Part model, mm, in its own coordinate system. Round coordinates to 2 decimals unless told otherwise and drop trailing zeros. Loops run counter-clockwise (first coordinate to the right, second up) from the corner with the lowest first, then second, coordinate; pieces in that order, holes last. Notation, with made-up numbers: M 44,42.25 L 67,42.25 A22 cw 67,62.25 Z; hole C -5,-18.5 d10. An arc over 180 degrees is marked long. Put each result on its own line as item: value. Start each with the question number.
1) Slice it at C-C on y = 155. Give the cut face in (x, z), then the cut area to 3 significant figures.
2) Probe line 1 along Y through (x, z) = (209, -2.25); line 2 along Y through (x, z) = (207.5, -1); line 3 along X through (y, z) = (99, 2.5). List the from-to ranges inside material, lowest first.
3) Pull direction X, two halves, no side cores. Call faces 1 (the cylindrical face through (212.715, 153.411, -0.07)), 2 (the cylindrical face through (215.896, 139.327, 0.07)), 3 (the flat face through (209, 140, -5)): +X half, -X half, draft (parallel to the pull), parting line (faces both ways), or undercut.
4) Slice it at D-D on y = 135.5. Give the cut face in (x, z), then the cut area to 3 significant figures.
5) Slice it at B-B on x = 208.5. Give the cut face in (y, z), then the cut area to 3 significant figures.
6) Slice it at A-A on z = 0.5. Give the cut face in (x, y) (3 decimals), then the cut area to 3 significant figures.
7) Drop flat-ended pins along their axis: pin 1 Ø1.5 at (x, z) = (203.5, -3) entering from +Y; pin 2 Ø2 at (x, z) = (201.5, 3.5) entering from +Y; pin 3 Ø1.5 at (x, z) = (214.5, -3) entering from -Y. Give the stop position or say it passes through.
```python
from build123d import *

# Parameters (mm, degrees)
ESBO_O1_R                = 4.15
ESBO_O1_R_2              = 5.175
RESSALTO_EXTRUS_O1_DEPTH = 5


with BuildPart() as part:
    # Esboço1 → Ressalto-extrusão1 (new, symmetric)
    with BuildSketch(Plane.XY):
        with BuildLine():
            ThreePointArc((198.88140452, 100), (208.88140452, 90), (218.88140452, 100))
            ThreePointArc((218.88140452, 100), (215.88140452, 139.886857429), (216.88140452, 179.873872767))
            ThreePointArc((216.88140452, 179.873872767), (208.88140452, 187.873872767), (200.88140452, 179.873872767))
            ThreePointArc((200.88140452, 179.873872767), (201.88140452, 139.886857429), (198.88140452, 100))
        make_face()
        with Locations((208.88140452, 155)):
            Circle(ESBO_O1_R, mode=Mode.SUBTRACT)
        with Locations((208.88140452, 179.873872767)):
            Circle(ESBO_O1_R, mode=Mode.SUBTRACT)
        with Locations((208.88140452, 100)):
            Circle(ESBO_O1_R_2, mode=Mode.SUBTRACT)
    extrude(amount=RESSALTO_EXTRUS_O1_DEPTH, both=True)


solid = part.part
```
Recorded:
1. outline: M 201.97,-5 L 204.73,-5 L 204.73,5 L 201.97,5 Z; M 213.03,-5 L 215.79,-5 L 215.79,5 L 213.03,5 Z
1. area: 55.1 mm2
2. line 1: y = 90 to 94.83, 105.17 to 150.85, 159.15 to 175.73, 184.02 to 187.87
2. line 2: y = 90.1 to 95.01, 104.99 to 151.09, 158.91 to 175.96, 183.79 to 187.75
2. line 3: x = 198.93 to 203.8, 213.96 to 218.83
3. face 1: undercut
3. face 2: +X half
3. face 3: draft
4. outline: M 201.75,-5 L 216.02,-5 L 216.02,5 L 201.75,5 Z
4. area: 143 mm2
5. outline: M 90.01,-5 L 94.84,-5 L 94.84,5 L 90.01,5 Z; M 105.16,-5 L 150.87,-5 L 150.87,5 L 105.16,5 Z; M 159.13,-5 L 175.74,-5 L 175.74,5 L 159.13,5 Z; M 184.01,-5 L 187.86,-5 L 187.86,5 L 184.01,5 Z
5. area: 710 mm2
6. outline: M 198.881,100 A10 ccw 218.881,100 A399.865 cw 216.881,179.874 A8 ccw 200.881,179.874 A399.865 cw Z; hole C 208.881,100 d10.35; hole C 208.881,155 d8.3; hole C 208.881,179.874 d8.3
6. area: 1,290 mm2
7. pin 1: stops at y = 186.4
7. pin 2: stops at y = 184.7
7. pin 3: stops at y = 91.27
